from build123d import *

# Parameters (mm, degrees)
SKETCH2_R           = 2.032
SKETCH2_W           = 65.0875
SKETCH2_H           = 203.2
BOSS_EXTRUDE1_DEPTH = 0.79375
SKETCH3_R           = 2.032
CUT_EXTRUDE1_DEPTH  = 223.550288208
FILLET1_R           = 9.525


with BuildPart() as part:
    # Sketch2 → Boss-Extrude1 (new, symmetric)
    with BuildSketch(Plane(origin=(0, 0, 0), x_dir=(1, 0, 0), z_dir=(0, 1, 0))):
        with BuildLine():
            Line((-51.59375, 58.370134809), (-128.507853241, 120.974637447))
            ThreePointArc((-128.507853241, 120.974637447), (-146.374637447, 119.142146759), (-144.542146759, 101.275362553))
            Line((-144.542146759, 101.275362553), (-51.59375, 25.619690772))
            Line((-51.59375, 25.619690772), (-51.59375, -25.619690772))
            Line((-51.59375, -25.619690772), (-144.542146759, -101.275362553))
            ThreePointArc((-144.542146759, -101.275362553), (-149.130906335, -112.668089589), (-141.929642552, -122.617599309))
            Line((-141.929642552, -122.617599309), (-51.59375, -165.1))
            Line((-51.59375, -165.1), (51.59375, -165.1))
            Line((51.59375, -165.1), (141.929642552, -122.617599309))
            ThreePointArc((141.929642552, -122.617599309), (149.130906335, -112.668089589), (144.542146759, -101.275362553))
            Line((144.542146759, -101.275362553), (51.59375, -25.619690772))
            Line((51.59375, -25.619690772), (51.59375, 25.619690772))
            Line((51.59375, 25.619690772), (144.542146759, 101.275362553))
            ThreePointArc((144.542146759, 101.275362553), (146.374637447, 119.142146759), (128.507853241, 120.974637447))
            Line((128.507853241, 120.974637447), (51.59375, 58.370134809))
            Line((51.59375, 58.370134809), (51.59375, 88.9))
            Line((51.59375, 88.9), (-51.59375, 88.9))
            Line((-51.59375, 88.9), (-51.59375, 58.370134809))
        make_face()
        with Locations(Location((-136.525, -111.125, 0), (0, 0, 270))):
            Circle(SKETCH2_R, mode=Mode.SUBTRACT)
        Polygon((-51.59375, -58.370134809), (-51.59375, -139.7), (-114.923666817, -109.917741521), align=None, mode=Mode.SUBTRACT)
        Polygon((51.59375, -139.7), (51.59375, -58.370134809), (114.923666817, -109.917741521), align=None, mode=Mode.SUBTRACT)
        with Locations(Location((136.525, -111.125, 0), (0, 0, 270))):
            Circle(SKETCH2_R, mode=Mode.SUBTRACT)
        with Locations((0, -38.1)):
            Rectangle(SKETCH2_W, SKETCH2_H, mode=Mode.SUBTRACT)
        with Locations(Location((-136.525, 111.125, 0), (0, 0, 270))):
            Circle(SKETCH2_R, mode=Mode.SUBTRACT)
        with Locations(Location((136.525, 111.125, 0), (0, 0, 270))):
            Circle(SKETCH2_R, mode=Mode.SUBTRACT)
    extrude(amount=BOSS_EXTRUDE1_DEPTH, both=True)

    # Sketch3 → Cut-Extrude1 (cut, through all)
    with BuildSketch(Plane.XZ.offset(0.79375)):
        with Locations(Location((44.45, 146.05, 0), (0, 0, 270))):
            Circle(SKETCH3_R)
        with Locations(Location((-44.45, 146.05, 0), (0, 0, 270))):
            Circle(SKETCH3_R)
        with Locations(Location((44.45, -69.85, 0), (0, 0, 270))):
            Circle(SKETCH3_R)
        with Locations(Location((-44.45, -69.85, 0), (0, 0, 270))):
            Circle(SKETCH3_R)
        with Locations(Location((-19.05, -69.85, 0), (0, 0, 270))):
            Circle(SKETCH3_R)
        with Locations(Location((19.05, -69.85, 0), (0, 0, 270))):
            Circle(SKETCH3_R)
        with Locations(Location((-19.05, -82.55, 0), (0, 0, 270))):
            Circle(SKETCH3_R)
        with Locations(Location((19.05, -82.55, 0), (0, 0, 270))):
            Circle(SKETCH3_R)
        with Locations(Location((-44.45, 36.180232558, 0), (0, 0, 270))):
            Circle(SKETCH3_R)
        with Locations(Location((44.45, 36.180232558, 0), (0, 0, 270))):
            Circle(SKETCH3_R)
    extrude(amount=-CUT_EXTRUDE1_DEPTH, mode=Mode.SUBTRACT)

    # Fillet1
    fillet1_edges = [part.edges().sort_by_distance(p)[0] for p in [
        (-51.59375, 0, 58.370134809),
        (-114.923666817, 0, 109.917741521),
        (-51.59375, 0, 139.7),
        (32.54375, 0, -63.5),
        (-32.54375, 0, -63.5),
        (-32.54375, 0, 139.7),
        (32.54375, 0, 139.7),
        (51.59375, 0, 58.370134809),
        (51.59375, 0, 139.7),
        (114.923666817, 0, 109.917741521),
        (-51.59375, 0, 25.619690772),
        (-51.59375, 0, -25.619690772),
        (-51.59375, 0, -58.370134809),
        (-51.59375, 0, -88.9),
        (51.59375, 0, -88.9),
        (51.59375, 0, -58.370134809),
        (51.59375, 0, -25.619690772),
        (51.59375, 0, 25.619690772),
        (51.59375, 0, 165.1),
        (-51.59375, 0, 165.1),
    ]]
    fillet(fillet1_edges, radius=FILLET1_R)


solid = part.part
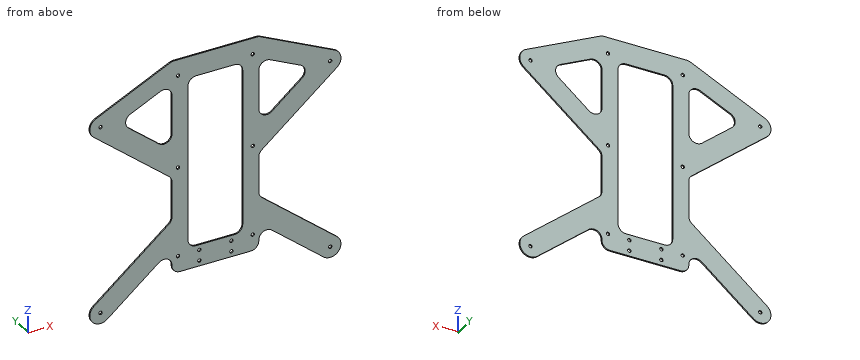
Design review of the part built by this model. Coordinates are the model's own, in mm. Coordinates: 2 decimals unless noted, no trailing zeros. Order: outer loops, then holes, each group sorted by start corner. A loop starts at its lowest first (then second) coordinate and runs counter-clockwise, first axis right, second up.
Item 1: Take a section at B-B, the plane z = 90.5. Write out the cut boundary in (x, y).
Item 2: For pin 1 Ø3.5 at (x, z) = (-44.45, -69.85) entering from +Y; pin 2 Ø0.5 at (y, z) = (0, 37) entering from -X; pin 3 Ø0.8 at (y, z) = (0.5, 7) entering from -X; pin 4 Ø0.8 at (y, z) = (0, -79) entering from +X, all flat-tipped, find the tip position at first contact; note any pin that passes through.
Item 3: Take a section at A-A, the plane x = -61.5. Write out the cut boundary in (y, z).
Item 4: Take a section at C-C, the plane y = -0.1. Count the separate pieces of the cut face and the enclosed holes in it, then the cut area to 3 significant figures.
Item 5: For line 1 (X direction, y = 0.3, z = 0.5); line 2 (Z direction, x = -20, y = -0.4); line 3 (X direction, y = -0.4, z = 130.5), list the stretches that pass through material, from the lowest coordinate up.
The answers:
1. outline: (-131.3, -0.79) - (-91.07, -0.79) - (-91.07, 0.79) - (-131.3, 0.79) - close; (-51.59, -0.79) - (-32.54, -0.79) - (-32.54, 0.79) - (-51.59, 0.79) - close; (32.54, -0.79) - (51.59, -0.79) - (51.59, 0.79) - (32.54, 0.79) - close; (91.07, -0.79) - (131.3, -0.79) - (131.3, 0.79) - (91.07, 0.79) - close
2. pin 1: passes through
2. pin 2: stops at x = -65.88
2. pin 3: stops at x = -51.59
2. pin 4: stops at x = 117.67
3. outline: (-0.79, -68.89) - (0.79, -68.89) - (0.79, -33.68) - (-0.79, -33.68) - close; (-0.79, 33.68) - (0.79, 33.68) - (0.79, 68.89) - (-0.79, 68.89) - close; (-0.79, 134.21) - (0.79, 134.21) - (0.79, 160.44) - (-0.79, 160.44) - close
4. separate pieces: 1
4. enclosed holes: 17
4. area: 29,300 mm2
5. line 1: x = -51.59 to -32.54, 32.54 to 51.59
5. line 2: z = -88.9 to -84.35, -80.75 to -71.65, -68.05 to -63.5, 139.7 to 165.1
5. line 3: x = -125.17 to -71.16, -53.57 to -32.54, 32.54 to 53.57, 71.16 to 125.17
